```python
from build123d import *

# Parameters (mm, degrees)
SKETCH1_W           = 36
SKETCH1_H           = 16
BOSS_EXTRUDE1_DEPTH = 165.35
SKEW_CUT_DEPTH      = 172.291046176


with BuildPart() as part:
    # Sketch1 → Boss-Extrude1 (new body)
    with BuildSketch(Plane.XY):
        with BuildLine():
            Line((0.2, 0), (39.8, 0))
            ThreePointArc((39.8, 0), (39.941421356, 0.058578644), (40, 0.2))
            Line((40, 0.2), (40, 19.8))
            ThreePointArc((40, 19.8), (39.941421356, 19.941421356), (39.8, 20))
            Line((39.8, 20), (0.2, 20))
            ThreePointArc((0.2, 20), (0.058578644, 19.941421356), (0, 19.8))
            Line((0, 19.8), (0, 0.2))
            ThreePointArc((0, 0.2), (0.058578644, 0.058578644), (0.2, 0))
        make_face()
        with Locations((20, 10)):
            Rectangle(SKETCH1_W, SKETCH1_H, mode=Mode.SUBTRACT)
    extrude(amount=BOSS_EXTRUDE1_DEPTH)

    # Sketch2 → Skew Cut (cut, through all)
    with BuildSketch(Plane.ZY):
        Polygon((0, 20), (34.641016151, 20), (0, 0), align=None)
        Polygon((165.35, 0), (153.802994616, 20), (165.35, 20), align=None)
    extrude(amount=-SKEW_CUT_DEPTH, mode=Mode.SUBTRACT)


solid = part.part
```
The model under review builds one solid part; all positions refer to its coordinate system, in mm. A direction names the side the tool comes from. Round coordinates to 2 decimals unless told otherwise and drop trailing zeros. Loops run counter-clockwise (first coordinate to the right, second up) from the corner with the lowest first, then second, coordinate; pieces in that order, holes last. Notation, with made-up numbers: M 16.5,-34 L 65.5,-34 A23 cw 65.5,-14 Z; hole C 84,-1.75 d5. An arc over 180 degrees is marked long. Put each result on its own line as item: value.
Q1. To check wall thickness, follow L1, parallel to Y at x = 37.5, z = 139.5; L2, parallel to X at y = 15.75, z = 34.5; L3, parallel to Y at x = 14, z = 157.5. State the ranges of each line that lie inside material, in increasing order.
Result set:
L1: y = 0 to 2, 18 to 20
L2: x = 0 to 2, 38 to 40
L3: y = 0 to 2
Q2. Consider section B-B, the plane x = 18.5. Give the boundary of the cut face in (y, z), then the cut area to 3 significant figures.
Result set:
outline: M 0,0 L 2,3.46 L 2,164.2 L 0,165.35 Z; M 18,31.18 L 20,34.64 L 20,153.8 L 18,154.96 Z
area: 569 mm²
Q3. Consider section A-A, the plane z = 117. Give the boundary of the cut face in (x, y).
Result set:
outline: M 0,0.2 A0.2 ccw 0.2,0 L 39.8,0 A0.2 ccw 40,0.2 L 40,19.8 A0.2 ccw 39.8,20 L 0.2,20 A0.2 ccw 0,19.8 Z; hole M 2,2 L 38,2 L 38,18 L 2,18 Z
Q4. Consider section D-D, the plane z = 22. Give the boundary of the cut face in (x, y).
Result set:
outline: M 0,0.2 A0.2 ccw 0.2,0 L 39.8,0 A0.2 ccw 40,0.2 L 40,12.7 L 38,12.7 L 38,2 L 2,2 L 2,12.7 L 0,12.7 Z
Q5. Machinability: for faces 5 (the flat face through (20, 2, 83)), 6 (the flat face through (20, 20, 93)), which of the approach directions +Z, -Z, +X, -X, +Y, -Y give a long, thin tool a straight path to every point of the face, cutting with its end or side? Answer none if there is none.
Result set:
face 5: +Z, -Z
face 6: +Z, -Z, +X, -X, +Y
Q6. Mouldability with a two-part tool opening along X and no side actions: class faces 1 (the flat face through (18.425, 1.805, 164.308)), 2 (the flat face through (0, 10, 82)), 3 (the flat face through (40, 10, 82)), 4 (the flat face through (20, 18, 92)) as released by +X, released by -X, zero draft, split by the parting line, or undercut.
Result set:
face 1: zero draft
face 2: released by -X
face 3: released by +X
face 4: undercut
Q7. Consider section C-C, the plane y = 3.5. Give the boundary of the cut face in (x, z).
Result set:
outline: M 0,6.06 L 2,6.06 L 2,163.33 L 0,163.33 Z; M 38,6.06 L 40,6.06 L 40,163.33 L 38,163.33 Z
